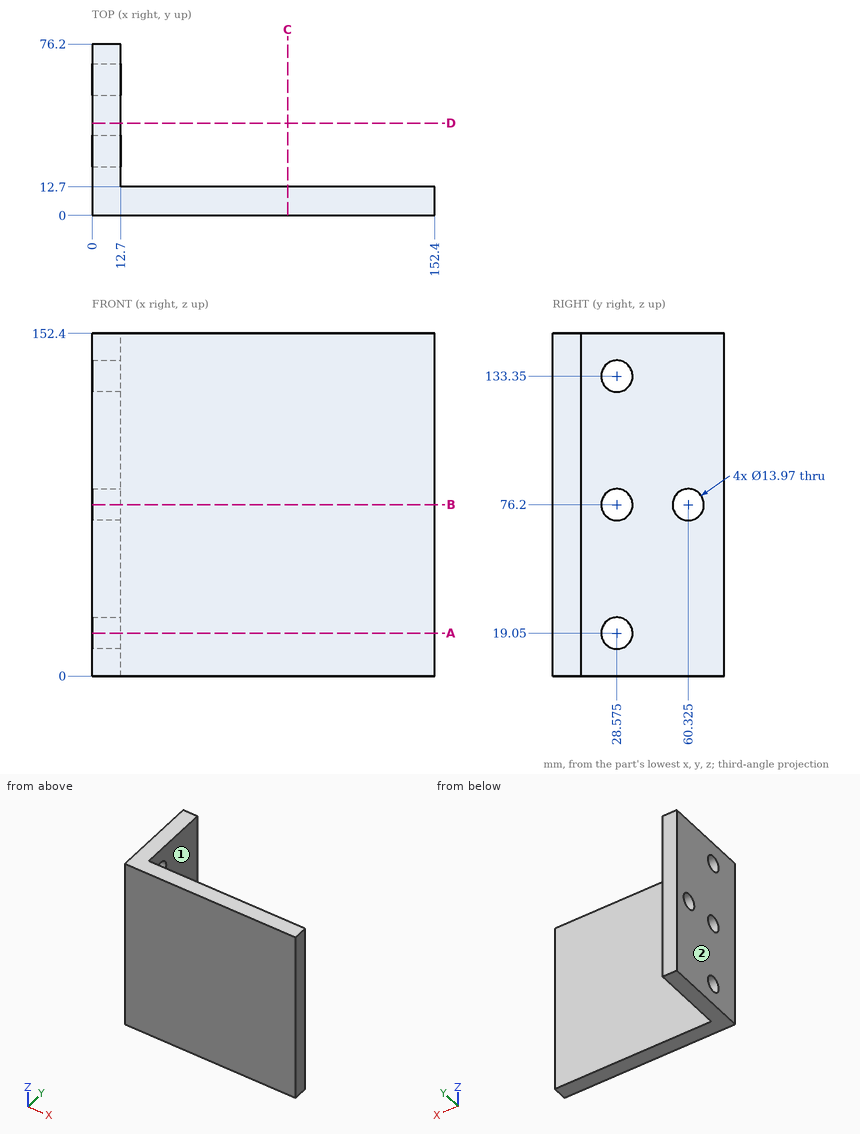
The figure shows three views and two pictorial views of one solid part (mm, origin at its lowest corner). Answer the questions. A direction names the side the tool comes from. Round coordinates to 2 decimals unless told otherwise and drop trailing zeros. Write each loop counter-clockwise with the first axis right and the second up, starting at its lowest first coordinate (ties: lowest second). Pieces come first, ordered by that corner, then holes. Notation, with made-up numbers: M 26,23.5 L 66,23.5 A7 cw 66,31.5 Z; hole C -33.5,46.25 d4. An arc over 180 degrees is marked long. Write each question's results on one line, items separated by ' | '. Start each with the question number.
(1) The part is cut by section C-C, the plane x = 87. Write down the section's boundary in (y, z), and give its area (3 significant figures).
(2) The part is cut by section A-A, the plane z = 19.05. Write down the section's boundary in (x, y), and give its area (3 significant figures).
(3) The part is cut by section B-B, the plane z = 76.2. Write down the section's boundary in (x, y).
(4) Each of these flat-tipped pins is pushed along its axis until it touches: P1, Ø16, axis at y = 28.575, z = 76.2, coming from the -X side; P2, Ø11, axis at y = 28.575, z = 19.05, coming from the -X side; P3, Ø5, axis at y = 16, z = 61, coming from the +X side. Where does it stop, or does it pass through?
(5) Find the intervals of material crossed by line 1 (Y direction, x = 7, z = 76); line 2 (X direction, y = 36.5, z = 145.5), in increasing order.
(6) For the marked faces 1 and 2, determine the directions among +Z, -Z, +X, -X, +Y, -Y from which every point of the face is accessible in a straight line to the end or side of a thin tool.
Worked answers:
1) outline: M 0,0 L 12.7,0 L 12.7,152.4 L 0,152.4 Z | area: 1,940 mm²
2) outline: M 0,0 L 152.4,0 L 152.4,12.7 L 12.7,12.7 L 12.7,21.59 L 0,21.59 Z; M 0,35.56 L 12.7,35.56 L 12.7,76.2 L 0,76.2 Z | area: 2,560 mm²
3) outline: M 0,0 L 152.4,0 L 152.4,12.7 L 12.7,12.7 L 12.7,21.59 L 0,21.59 Z; M 0,35.56 L 12.7,35.56 L 12.7,53.34 L 0,53.34 Z; M 0,67.31 L 12.7,67.31 L 12.7,76.2 L 0,76.2 Z
4) P1: stops at x = 0 | P2: passes through | P3: stops at x = 12.7
5) line 1: y = 0 to 21.59, 35.56 to 53.34, 67.31 to 76.2 | line 2: x = 0 to 12.7
6) face 1: +Z, -Z, +X, +Y | face 2: +Z, -Z, -X, +Y, -Y
